from build123d import *

# Parameters (mm, degrees)
F0_W     = 125
F0_H     = 75
F1_DEPTH = 37.5
F2_W     = 105
F2_H     = 30
F3_DEPTH = 75
F5_START = 50
F4_W     = 70
F4_H     = 45
F5_DEPTH = 32.67132
F6_W     = 27.5
F6_H     = 15
F7_DEPTH = 50
F8_W     = 35
F8_H     = 10
F9_DEPTH = 79.66762


with BuildPart() as f1:
    # F0 (on Front) → F1 (new body, symmetric)
    with BuildSketch(Plane.XZ):
        with Locations((-0.445794413, 37.5)):
            Rectangle(F0_W, F0_H)
    extrude(amount=F1_DEPTH, both=True)

    # F2 (on Top) → F3 (cut, symmetric)
    with BuildSketch(Plane.XY):
        with Locations((-10.445794413, -22.5)):
            Rectangle(F2_W, F2_H)
    extrude(amount=F3_DEPTH, both=True, mode=Mode.SUBTRACT)

    # F4 (on Top) → F5 (cut)
    with BuildSketch(Plane.XY.offset(F5_START)):
        with Locations((-2.945794413, 15)):
            Rectangle(F4_W, F4_H)
    extrude(amount=F5_DEPTH, mode=Mode.SUBTRACT)

    # F6 (on Top) → F7 (cut, symmetric)
    with BuildSketch(Plane.XY):
        with Locations((-6.695794413, 0)):
            Rectangle(F6_W, F6_H)
    extrude(amount=F7_DEPTH, both=True, mode=Mode.SUBTRACT)

    # F8 (on Top) → F9 (cut)
    with BuildSketch(Plane.XY):
        with Locations((24.554205587, -2.5)):
            Rectangle(F8_W, F8_H)
    extrude(amount=F9_DEPTH, mode=Mode.SUBTRACT)


solid = f1.part
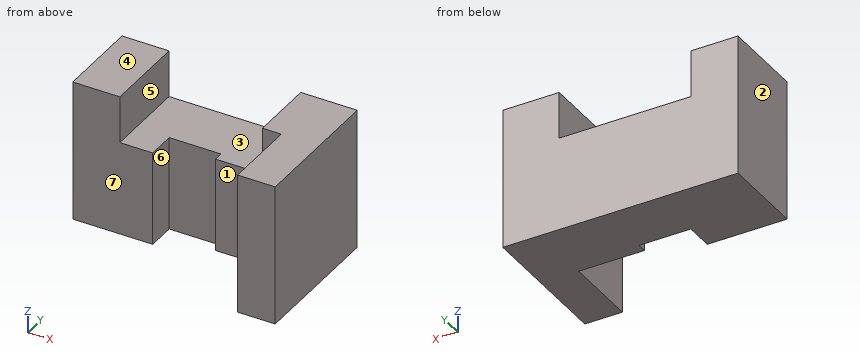
Part model, mm, in its own coordinate system. Face numbers are marked on the shaded views. A direction names the side the tool comes from. Round coordinates to 2 decimals unless told otherwise and drop trailing zeros. Write each loop counter-clockwise with the first axis right and the second up, starting at its lowest first coordinate (ties: lowest second). Pieces come first, ordered by that corner, then holes. Notation, with made-up numbers: (63, 49) - (81, 49) arc R25 ccw to (81, 87) - close; hole circle Ø3 at (28, 72.25). An arc over 180 degrees is marked (long way). Use CSV: the item, a comma, the result in double quotes.
Item 1: Pull direction X, two halves, no side cores. Call the marked faces 1, 2, 3 and 4: pulls with the +X half, pulls with the -X half, needs draft (parallel to the pull), parting line crosses it, or undercut.
Results list:
face 1,"undercut"
face 2,"pulls with the -X half"
face 3,"undercut"
face 4,"needs draft"
Item 2: Slice it at B-B, the plane y = 17. Write the cut outline in (x, z).
Results list:
outline,"(-62.95, 0) - (62.05, 0) - (62.05, 75) - (32.05, 75) - (32.05, 50) - (-37.95, 50) - (-37.95, 75) - (-62.95, 75) - close"
Item 3: Tool access for the marked faces 5, 6 and 7: list every direction of +Z, -Z, +X, -X, +Y, -Y with a clear straight run to the whole face (end or side of a thin tool).
Results list:
face 5,"+Z, +Y, -Y"
face 6,"+Z, -Z, -Y"
face 7,"+Z, -Z, -X, -Y"
Item 4: Slice it at D-D, the plane x = 12. Write the cut outline in (y, z).
Results list:
outline,"(2.5, 0) - (37.5, 0) - (37.5, 50) - (2.5, 50) - close"
Item 5: Slice it at A-A, the plane z = 65. Write the cut outline in (x, y), then the cut area to 4 significant figures.
Results list:
outline,"(-62.95, -7.5) - (-37.95, -7.5) - (-37.95, 37.5) - (-62.95, 37.5) - close; (32.05, 2.5) - (42.05, 2.5) - (42.05, -37.5) - (62.05, -37.5) - (62.05, 37.5) - (32.05, 37.5) - close"
area,"2,975 mm²"
Item 6: Flat gauge pins, fed straight in: P1, Ø3, axis at x = 44, y = -6.5, coming from the -Z side; P2, Ø4, axis at x = -43.5, z = 65.5, coming from the -Y side; P3, Ø10.5, axis at x = 20, z = 21, coming from the -Y side; P4, Ø8, axis at x = -9, z = 28, coming from the -Y side. Where does each tip first touch, or does it go through?
Results list:
P1,"stops at z = 0"
P2,"stops at y = -7.5"
P3,"stops at y = 2.5"
P4,"stops at y = 7.5"
Item 7: Wall check: L1, parallel to X at y = -2, z = 13; L2, parallel to X at y = 5, z = 33.5; L3, parallel to Y at x = -54, z = 57. Give the ranges that are in metal, low to high.
Results list:
L1,"x = -62.95 to -20.45, 42.05 to 62.05"
L2,"x = -62.95 to -20.45, 7.05 to 62.05"
L3,"y = -7.5 to 37.5"
Item 8: Slice it at C-C, the plane z = 38. Write the cut outline in (x, y).
Results list:
outline,"(-62.95, -7.5) - (-20.45, -7.5) - (-20.45, 7.5) - (7.05, 7.5) - (7.05, 2.5) - (42.05, 2.5) - (42.05, -37.5) - (62.05, -37.5) - (62.05, 37.5) - (-62.95, 37.5) - close"
